The drawing under review shows one solid part. Ordinate dimensions are in mm from its lowest x, y, z. A direction names the side the tool comes from. Round coordinates to 2 decimals unless told otherwise and drop trailing zeros. Write each loop counter-clockwise with the first axis right and the second up, starting at its lowest first coordinate (ties: lowest second). Pieces come first, ordered by that corner, then holes. Notation, with made-up numbers: M 80.5,-35 L 87.5,-35 A36 ccw 87.5,3 Z; hole C 31,-21.5 d9. An arc over 180 degrees is marked long. One line per item, written item: value. Start each with the question number.
1) For P1, Ø1, axis at y = 4.5, z = 12, coming from the +X side; P2, Ø1.5, axis at x = 11.5, y = 2, coming from the +Z side, all flat-tipped, find the tip position at first contact; note any pin that passes through.
2) Tool access review of the marked faces 5 and 6: name each direction out of +Z, -Z, +X, -X, +Y, -Y from which nothing blocks a thin tool from reaching the whole face with its end or side.
3) Take a section at D-D, the plane x = 29. Write out the cut boundary in (y, z), and give its area (3 significant figures).
4) Mouldability with a two-part tool opening along X and no side actions: class the marked faces 1, 2, 3 and 4 as +X half, -X half, draft (parallel to the pull), parting line (faces both ways), or undercut.
5) Take a section at B-B, the plane x = 2. Write out the cut boundary in (y, z), and give its area (3 significant figures).
6) Take a section at C-C, the plane y = 1.6. Write out the cut boundary in (x, z), and give its area (3 significant figures).
7) Wall thickness on probe 1 along Z at (x, y) = (18.5, 2.15); probe 2 along X at (y, z) = (3.25, 14.5); probe 3 along X at (y, z) = (4, 10.25): over which ranges is each line inside the solid? List them lowest first.
8) Take a section at A-A, the plane z = 11.25. Write out the cut boundary in (x, y), and give its area (3 significant figures).
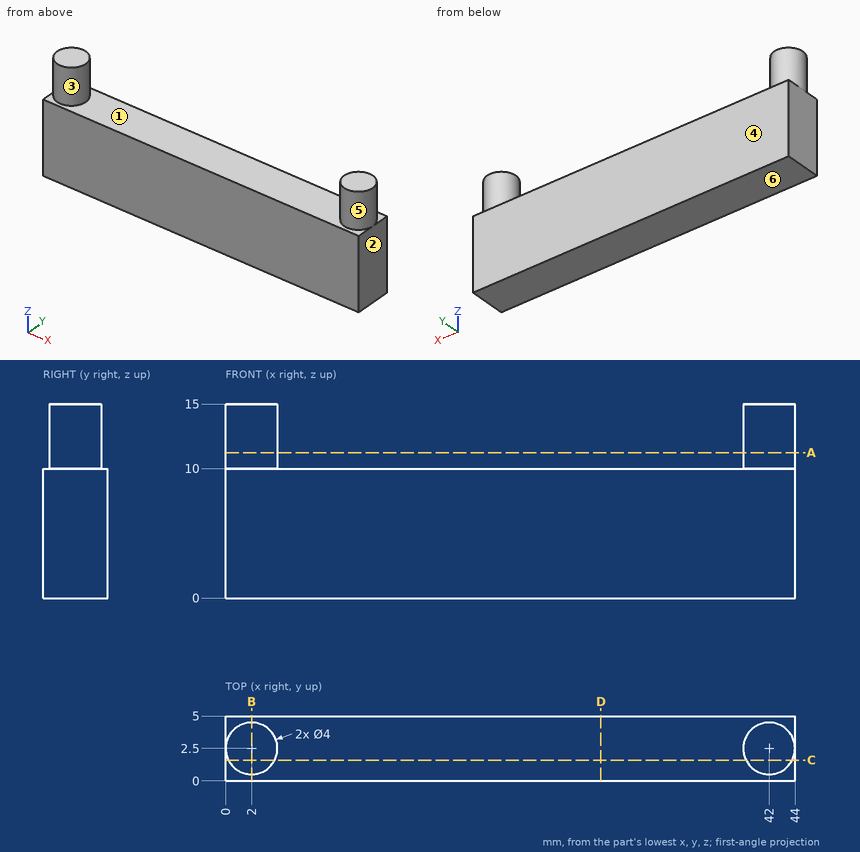
Checked values:
1. P1: stops at x = 43.32
1. P2: stops at z = 10
2. face 5: +Z
2. face 6: -Z, +X, -X, +Y, -Y
3. outline: M 0,0 L 5,0 L 5,10 L 0,10 Z
3. area: 50.0 mm2
4. face 1: undercut
4. face 2: +X half
4. face 3: undercut
4. face 4: draft
5. outline: M 0,0 L 5,0 L 5,10 L 4.5,10 L 4.5,15 L 0.5,15 L 0.5,10 L 0,10 Z
5. area: 70.0 mm2
6. outline: M 0,0 L 44,0 L 44,10 L 43.79,10 L 43.79,15 L 40.21,15 L 40.21,10 L 3.79,10 L 3.79,15 L 0.21,15 L 0.21,10 L 0,10 Z
6. area: 476 mm2
7. probe 1: z = 0 to 10
7. probe 2: x = 0.15 to 3.85, 40.15 to 43.85
7. probe 3: x = 0.68 to 3.32, 40.68 to 43.32
8. outline: C 2,2.5 d4; C 42,2.5 d4
8. area: 25.1 mm2
